Autodesk Inventor part; units mm, degrees
ref_plane "YZ Plane" through (0, 0, 0) normal (1, 0, 0) x (0, 1, 0)
ref_plane "XZ Plane" through (0, 0, 0) normal (0, 1, 0) x (-1, 0, 0)
ref_plane "XY Plane" through (0, 0, 0) normal (0, 0, 1) x (1, 0, 0)
sketch "Sketch1" plane through (0, 0, 0) normal (0, 0, 1) x (1, 0, 0)
  line L0 (0, 0) -> (25, 0)
  line L1 (25, 0) -> (25, 40)
  line L2 (25, 40) -> (0, 40)
  line L3 (0, 40) -> (0, 0)
  dimension "d1" = 25
  dimension "d2" = 40
  dimension "d3" = 25
extrude "Extrusion1" add sketch "Sketch1" against normal blind 30
sketch "Sketch2" plane through (25, 0, 0) normal (1, 0, 0) x (0, 0, -1)
  line L0 (0, 0) -> (30, 0)
  circle A0 centre (15, 6.56) radius 2.46
extrude "Extrusion2" cut sketch "Sketch2" against normal blind 30
sketch "Sketch3" plane through (0, 0, 0) normal (-1, 0, 0) x (0, 0, 1)
  line L0 (0, 0) -> (-30, 0)
  line L1 (-25.05, 0) -> (-4.95, 0)
  line L2 (-4.95, 0) -> (-4.95, 33.12)
  line L3 (-4.95, 33.12) -> (-25.05, 33.12)
  line L4 (-25.05, 33.12) -> (-25.05, 0)
  dimension "d11" = 20.1
extrude "Extrusion3" cut sketch "Sketch3" against normal blind 20
sketch "Sketch4" plane through (0, 0, 0) normal (0, -1, 0) x (1, 0, 0)
  line L0 (20, -4.95) -> (20, -25.05)
  line L1 (20, -15) -> (25, -15)
  line L2 (25, 0) -> (25, -30)
  line L3 (20, -8.025) -> (25, -8.025)
  line L4 (25, -8.025) -> (25, -21.975)
  line L5 (25, -21.975) -> (20, -21.975)
  line L6 (20, -21.975) -> (20, -8.025)
  line L7 (20, -8.025) -> (25, -21.975) construction
  line L8 (25, -8.025) -> (20, -21.975) construction
  line L9 (25, -12.54) -> (25, -17.46)
  point P0 (0, 0)
  point P1 (22.5, -15)
  dimension "d14" = 13.95
extrude "Extrusion4" add sketch "Sketch4" along normal blind 15
sketch "Sketch5" plane through (20, 0, 0) normal (-1, 0, 0) x (0, 0, 1)
  circle A0 centre (-15, 6.56) radius 2.46
  circle A1 centre (-15, 6.56) radius 4.7025
  circle A2 centre (-15, 6.56) radius 2.46
  circle A3 centre (-15, 6.56) radius 2.46
  point P0 (0, 0)
  dimension "d17" = 9.405
extrude "Extrusion5" cut sketch "Sketch5" against normal blind 2.1
sketch "Sketch6" plane through (25, 0, 0) normal (1, 0, 0) x (0, 0, -1)
  circle A0 centre (15, 6.56) radius 4.7025
  line L0 (15, 6.56) -> (15, 23.56)
  circle A1 centre (15, 23.56) radius 2.46
  point P0 (0, 0)
  dimension "d20" = 17
  dimension "d21" = 4.92
extrude "Extrusion6" cut sketch "Sketch6" against normal blind 10 contours A1
sketch "Sketch7" plane through (20, 0, 0) normal (-1, 0, 0) x (0, 0, 1)
  circle A0 centre (-15, 23.56) radius 2.46
  circle A1 centre (-15, 23.56) radius 4.7025
  point P0 (0, 0)
  dimension "d24" = 9.405
extrude "Extrusion7" cut sketch "Sketch7" against normal blind 2.1
sketch "Sketch9" plane through (25, 0, 0) normal (1, 0, 0) x (0, 0, -1)
  circle A0 centre (15, 6.56) radius 2.46
  circle A1 centre (15, 6.56) radius 2.46
  circle A2 centre (15, 23.56) radius 2.46
  circle A3 centre (15, 23.56) radius 2.46
  line L0 (30, 40) -> (30, 0)
  line L1 (30, 0) -> (30, 40)
  line L2 (30, 40) -> (0, 40)
  line L3 (0, 40) -> (0, 0)
  line L4 (0, 0) -> (8.025, 0)
  line L5 (21.975, 0) -> (21.975, -15)
  line L6 (21.975, -15) -> (8.025, -15)
  line L7 (8.025, -15) -> (8.025, 0)
  line L8 (0, 0) -> (8.025, 0)
  line L9 (21.975, 0) -> (30, 0)
extrude "Extrusion8" add sketch "Sketch9" along normal blind 5
sketch "Sketch10" plane through (0, 40, 0) normal (0, 1, 0) x (1, 0, 0)
  line L0 (0, 30) -> (30, 30)
  line L1 (30, 0) -> (0, 0)
  line L2 (0, 30) -> (30, 30)
  line L3 (30, 30) -> (30, 0)
  line L4 (30, 0) -> (0, 0)
  line L5 (0, 0) -> (0, 30)
extrude "Extrusion9" add sketch "Sketch10" along normal blind 30
sketch "Sketch12" plane through (30, 0, 0) normal (1, 0, 0) x (0, 0, -1)
  circle A0 centre (15, 6.56) radius 2.46
  line L0 (15, 6.56) -> (15, 15.06)
  circle A1 centre (15, 15.06) radius 2.525
  point P0 (0, 0)
  dimension "d31" = 8.5
  dimension "d33" = 5.05
extrude "Extrusion10" cut sketch "Sketch12" against normal blind 30 contours A1
sketch "Sketch14" plane through (0, 0, 0) normal (0, 0, 1) x (1, 0, 0)
  line L0 (30, 70) -> (0, 70)
  line L1 (0, 100) -> (-8, 100)
  line L2 (30, 0) -> (30, 70)
  line L3 (30, 118) -> (30, 70)
  line L4 (30, 105) -> (30, 100)
  line L5 (0, 70) -> (30, 70)
  line L6 (0, 70) -> (0, 100)
  line L7 (-8, 145) -> (15, 145)
  line L8 (-2, 142.5) -> (-8, 145)
  line L9 (-2, 102.5) -> (-8, 100)
  line L10 (-2, 102.5) -> (4, 122.5)
  line L11 (4, 122.5) -> (-2, 142.5)
  line L12 (15, 145) -> (30, 122.5)
  line L13 (30, 122.5) -> (30, 118)
  point P0 (0, 0)
  dimension "d47" = 30
  dimension "d85" = 45
extrude "Extrusion12" add sketch "Sketch14" against normal blind 30
sketch "Sketch15" plane through (0, 0, -25.05) normal (-1, 0, 0) x (0, 0, 1)
  line L0 (0, 33.12) -> (20.1, 33.12)
  line L1 (20.1, 33.12) -> (20.1, 0)
  line L2 (0, 33.12) -> (20.1, 33.12)
  line L3 (20.1, 33.12) -> (20.1, 31.1)
  line L4 (20.1, 31.1) -> (0, 31.1)
  line L5 (0, 31.1) -> (0, 33.12)
  point P0 (25.05, 0)
  dimension "d57" = 2.02
extrude "Extrusion13" add sketch "Sketch15" against normal blind 20
properties part number "40mm_x_30mm"
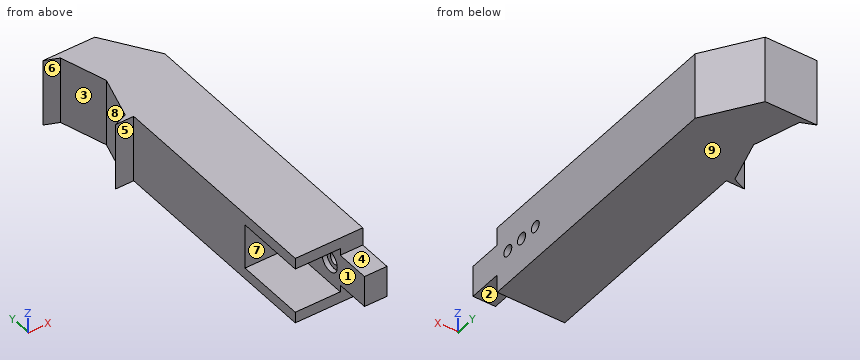
CAD build for the part. Positions are in the model's coordinates, mm. Face numbers are marked on the shaded views. A direction names the side the tool comes from. Give positions to 0.01 mm unless a question says otherwise; leave off trailing zeros. Write each loop counter-clockwise with the first axis right and the second up, starting at its lowest first coordinate (ties: lowest second). Pieces come first, ordered by that corner, then holes. Notation, with made-up numbers: M 39,75 L 88,75 A34 ccw 88,113 Z; hole C 73.25,19.5 d2. An arc over 180 degrees is marked long. Return JSON: item names as keys, results as strings. Group by question number.
(1) Band-saw the part on A-A (z = -15). State how many separate pieces and enclosed holes the cut face has, and give its area (3 significant figures).
(2) Band-saw the part on D-D (x = 9). Give the cut face in (y, z), and give its area (3 significant figures).
(3) Flat gauge pins, fed straight in: pin 1 Ø9 at (x, z) = (-5, -14.5) entering from -Y; pin 2 Ø15 at (y, z) = (23.56, -15) entering from -X; pin 3 Ø6 at (y, z) = (115.5, -18.5) entering from -X. Where does each tip first touch, or does it go through?
(4) Mould opens along Y. For the marked faces 6, 7, 8 and 9 say: pulls with the +Y half, pulls with the -Y half, needs draft (parallel to the pull), parting line crosses it, or undercut.
(5) Band-saw the part on B-B (x = 23.5). Give the cut face in (y, z) (3 decimals), and give its area (3 significant figures).
(6) Drill centre lines: L1, parallel to Z at x = 25, y = 15.06 (3 decimals); L2, parallel to Z at x = 12.5, y = 18.5; L3, parallel to Y at x = 27.25, z = -15 (3 decimals). Where is each one in solid material? Low to high. Write a range as [from, to].
(7) Band-saw the part on C-C (y = 6.56). Give the cut face in (x, z).
(8) 3-axis set-ups, long thin cutter, end or side, ignore diameter. For the marked faces 1, 2, 3, 4 and 5: which of +Z, -Z, +X, -X, +Y, -Y reach the whole face in a straight line?
Entries:
{
 "1": {"separate pieces": "4", "enclosed holes": "0", "area": "3,530 mm^2"},
 "2": {"outline": "M 0,-30 L 145,-30 L 145,0 L 0,0 L 0,-4.95 L 31.1,-4.95 L 31.1,-25.05 L 0,-25.05 Z", "area": "3,720 mm^2"},
 "3": {"pin 1": "stops at y = 100", "pin 2": "stops at x = 20", "pin 3": "stops at x = 1"},
 "4": {"face 6": "undercut", "face 7": "pulls with the -Y half", "face 8": "undercut", "face 9": "needs draft"},
 "5": {"outline": "M -15,-21.975 L 0,-21.975 L 0,-30 L 132.25,-30 L 132.25,0 L 0,0 L 0,-8.025 L -15,-8.025 Z; hole C 6.56,-15 d4.92; hole C 15.06,-15 d5.05; hole C 23.56,-15 d4.92", "area": "4,120 mm^2"},
 "6": {"L1": "z = [-30, -17.525], [-12.475, 0]", "L2": "z = [-30, -25.05], [-4.95, 0]", "L3": "y = [-15, 4.1], [9.02, 12.535], [17.585, 21.1], [26.02, 126.625]"},
 "7": {"outline": "M 0,-30 L 30,-30 L 30,-17.46 L 22.1,-17.46 L 22.1,-19.7 L 20,-19.7 L 20,-25.05 L 0,-25.05 Z; M 0,-4.95 L 20,-4.95 L 20,-10.3 L 22.1,-10.3 L 22.1,-12.54 L 30,-12.54 L 30,0 L 0,0 Z"},
 "8": {"face 1": "-X, -Y", "face 2": "-Z, +X, -X, -Y", "face 3": "+Z, -Z, -X", "face 4": "+Z, +X, -X, -Y", "face 5": "+Z, -Z, -X, -Y"}
}
